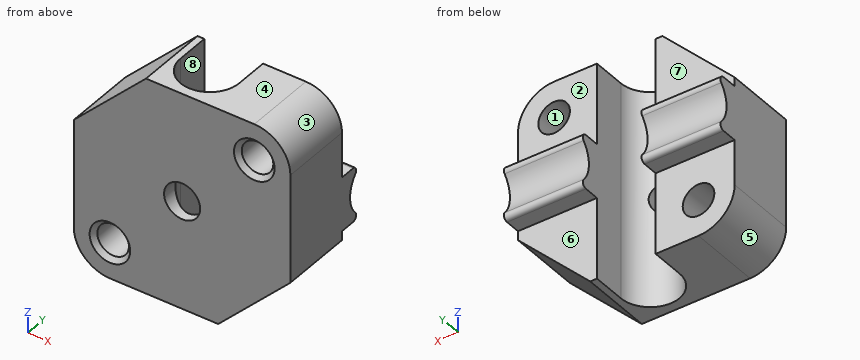
```python
from build123d import *

# Parameters (mm, degrees)
SKETCH_1_W               = 24
SKETCH_1_H               = 24
EXTRUDE_1_DEPTH          = 8
SKETCH_2_R               = 3.25
SKETCH_2_W               = 6.5
SKETCH_2_H               = 3.7
CUT_EXTRUDE_1_DEPTH      = 1
CUT_EXTRUDE_1_DEPTH_BACK = 25
EXTRUDE_2_DEPTH          = 8.75
SKETCH_5_R               = 1.75
CUT_EXTRUDE_3_DEPTH      = 9
CHAMFER_1_SIZE           = 8
FILLET_1_R               = 4
FILLET_2_R               = 0.5
SKETCH_9_R               = 2
CUT_EXTRUDE_4_DEPTH      = 11.204915028
CHAMFER_3_SIZE           = 0.5


with BuildPart() as part:
    # 草图1 → 凸台-拉伸1 (new body)
    with BuildSketch(Plane(origin=(0, 0, 0), x_dir=(1, 0, 0), z_dir=(0, 1, 0))):
        Rectangle(SKETCH_1_W, SKETCH_1_H)
    extrude(amount=EXTRUDE_1_DEPTH)

    # 草图2 → 切除-拉伸1 (cut, two sides)
    with BuildSketch(Plane.XY.offset(12)) as cut_extrude_1_sk:
        with Locations((0, 4.3)):
            Circle(SKETCH_2_R)
        with Locations((0, 6.15)):
            Rectangle(SKETCH_2_W, SKETCH_2_H)
    extrude(amount=CUT_EXTRUDE_1_DEPTH, mode=Mode.SUBTRACT)
    extrude(cut_extrude_1_sk.sketch, amount=-CUT_EXTRUDE_1_DEPTH_BACK, mode=Mode.SUBTRACT)

    # 草图4 → 凸台-拉伸2 (add)
    with BuildSketch(Plane(origin=(12, 0, 0), x_dir=(0, 0, -1), z_dir=(1, 0, 0))):
        with BuildLine():
            Line((-3, 8), (3, 8))
            Line((3, 8), (3, 11.25))
            ThreePointArc((3, 11.25), (0, 9.25), (-3, 11.25))
            Line((-3, 11.25), (-3, 8))
        make_face()
    extrude_2 = extrude(amount=-EXTRUDE_2_DEPTH)

    # 镜向2: 凸台-拉伸2 across plane
    add(extrude_2.mirror(Plane(origin=(0, 0, 0), x_dir=(0, 0, 1), z_dir=(1, 0, 0))))

    # 草图5 → 切除-拉伸3 (cut, through all)
    with BuildSketch(Plane(origin=(0, 8, 0), x_dir=(1, 0, 0), z_dir=(0, 1, 0))):
        with Locations((-8, 8)):
            Circle(SKETCH_5_R)
        with Locations((8, -8)):
            Circle(SKETCH_5_R)
    extrude(amount=-CUT_EXTRUDE_3_DEPTH, mode=Mode.SUBTRACT)

    # 倒角1
    chamfer_1_edges = [part.edges().sort_by_distance(p)[0] for p in [
        (-12, 4, 12),
        (12, 4, -12),
    ]]
    chamfer(chamfer_1_edges, length=CHAMFER_1_SIZE)

    # 圆角1
    fillet_1_edges = [part.edges().sort_by_distance(p)[0] for p in [
        (12, 4, 12),
        (-12, 4, -12),
    ]]
    fillet(fillet_1_edges, radius=FILLET_1_R)

    # 圆角2
    fillet_2_edges = [part.edges().sort_by_distance(p)[0] for p in [
        (7.625, 11.25, 3),
        (7.625, 11.25, -3),
        (-7.625, 11.25, -3),
        (-7.625, 11.25, 3),
    ]]
    fillet(fillet_2_edges, radius=FILLET_2_R)

    # 草图9 → 切除-拉伸4 (cut, through all)
    with BuildSketch(Plane.XZ):
        Circle(SKETCH_9_R)
    extrude(amount=-CUT_EXTRUDE_4_DEPTH, mode=Mode.SUBTRACT)

    # 倒角3
    chamfer_3_edges = [part.edges().sort_by_distance(p)[0] for p in [
        (-9.75, 0, -8),
        (6.25, 0, 8),
    ]]
    chamfer(chamfer_3_edges, length=CHAMFER_3_SIZE)


solid = part.part
```
Work out the finished part from the listing and answer in its coordinate system (mm). Face numbers are marked on the shaded views. A direction names the side the tool comes from. Round coordinates to 2 decimals unless told otherwise and drop trailing zeros. Order: outer loops, then holes, each group sorted by start corner. A loop starts at its lowest first (then second) coordinate and runs counter-clockwise, first axis right, second up.
Q1. Find the intervals of material crossed by line 1 along X through (y, z) = (6, -8); line 2 along X through (y, z) = (5.75, 8); line 3 along Z through (x, y) = (8, 3.5), in increasing order.
Solution:
line 1: x = -12 to -9.75, -6.25 to -3.25, 3.25 to 8
line 2: x = -8 to -3.25, 3.25 to 6.25, 9.75 to 12
line 3: z = -8 to 6.25, 9.75 to 12
Q2. The mould has two halves that part along X. Classify the marked faces 1, 2 and 3: pulls with the +X half, pulls with the -X half, needs draft (parallel to the pull), parting line crosses it, or undercut.
Solution:
face 1: undercut
face 2: needs draft
face 3: pulls with the +X half
Q3. A tool of negligible diameter and unlimited length cuts with its end or side. For the marked faces 4, 5, 6, 7 and 8, from which of +Z, -Z, +X, -X, +Y, -Y can it reach the whole face along a straight path? Write none if from no direction.
Solution:
face 4: +Z, +X, -X, +Y, -Y
face 5: -Z, -X, +Y, -Y
face 6: -Z, +X, -X, +Y
face 7: +Z, +X, -X, +Y
face 8: +Z, -Z, +Y
Q4. A cutting plane is placed at C-C, the plane x = 0.5. Determine the outline of the cut face in (y, z).
Solution:
outline: (0, -12) - (1.09, -12) - (1.09, -1.94) - (0, -1.94) - close; (0, 1.94) - (1.09, 1.94) - (1.09, 12) - (0, 12) - close
Q5. A cutting plane is placed at B-B, the plane z = -0.5. Determine the outline of the cut face in (x, y).
Solution:
outline: (-12, 0) - (-1.94, 0) - (-1.94, 1.69) arc R3.25 cw to (-3.25, 4.3) - (-3.25, 9.29) - (-12, 9.29) - close; (1.94, 0) - (12, 0) - (12, 9.29) - (3.25, 9.29) - (3.25, 4.3) arc R3.25 cw to (1.94, 1.69) - close
Q6. A cutting plane is placed at A-A, the plane y = 3.25. Determine the outline of the cut face in (x, z).
Solution:
outline: (-12, -8) arc R4 ccw to (-8, -12) - (-3.08, -12) - (-3.08, 12) - (-4, 12) - (-12, 4) - close; (3.08, -12) - (4, -12) - (12, -4) - (12, 8) arc R4 ccw to (8, 12) - (3.08, 12) - close; hole circle Ø3.5 at (-8, -8); hole circle Ø3.5 at (8, 8)
Q7. Given pin 1 Ø9.5 at (x, z) = (7, -8.5) entering from +Y; pin 2 Ø1.9 at (x, y) = (9, 8.5) entering from -Z; pin 3 Ø1.4 at (x, y) = (-8, 9) entering from -Z, each flat-ended and moving along its own axis, determine where each tip first touches the part or whether it passes through.
Solution:
pin 1: stops at y = 8
pin 2: stops at z = -7.81
pin 3: stops at z = -3
